from build123d import *

# Parameters (mm, degrees)
SKETCH1_R           = 8.743447226
SKETCH1_R_2         = 3
SKETCH1_R_3         = 10.172294787
SKETCH1_W           = 3
SKETCH1_H           = 12
BOSS_EXTRUDE1_DEPTH = 5
FILLET3_R           = 20
FILLET4_R           = 20
FILLET5_R           = 20


with BuildPart() as part:
    # Sketch1 → Boss-Extrude1 (new body)
    with BuildSketch(Plane(origin=(0, 0, 0), x_dir=(1, 0, 0), z_dir=(0, 1, 0))):
        Polygon((25, 35), (125, 35), (125, 111), (122, 111), (122, 123), (125, 123), (125, 175), (150, 175), (150, 200), (0, 200), (0, 175), (25, 175), (25, 123), (28, 123), (28, 111), (25, 111), align=None)
        with Locations(Location((75, 139.799864951, 0), (0, 0, 270))):
            Circle(SKETCH1_R, mode=Mode.SUBTRACT)
        with Locations(Location((93.745998674, 100, 0), (0, 0, 270))):
            Circle(SKETCH1_R_2, mode=Mode.SUBTRACT)
        with Locations(Location((93.745998674, 63.5, 0), (0, 0, 270))):
            Circle(SKETCH1_R_2, mode=Mode.SUBTRACT)
        with Locations(Location((75, 80.674864151, 0), (0, 0, 270))):
            Circle(SKETCH1_R_3, mode=Mode.SUBTRACT)
        with Locations(Location((57.245998674, 63.5, 0), (0, 0, 270))):
            Circle(SKETCH1_R_2, mode=Mode.SUBTRACT)
        with Locations(Location((57.245998674, 100, 0), (0, 0, 270))):
            Circle(SKETCH1_R_2, mode=Mode.SUBTRACT)
        with Locations((48, 117)):
            Rectangle(SKETCH1_W, SKETCH1_H, mode=Mode.SUBTRACT)
        with Locations(Location((45.771721368, 146.237160755, 0), (0, 0, 270))):
            Circle(SKETCH1_R_2, mode=Mode.SUBTRACT)
        with Locations(Location((45.771721368, 169.237160755, 0), (0, 0, 270))):
            Circle(SKETCH1_R_2, mode=Mode.SUBTRACT)
        with Locations((102, 117)):
            Rectangle(SKETCH1_W, SKETCH1_H, mode=Mode.SUBTRACT)
        with Locations(Location((103.771721368, 146.237160755, 0), (0, 0, 270))):
            Circle(SKETCH1_R_2, mode=Mode.SUBTRACT)
        with Locations(Location((103.771721368, 169.237160755, 0), (0, 0, 270))):
            Circle(SKETCH1_R_2, mode=Mode.SUBTRACT)
    extrude(amount=BOSS_EXTRUDE1_DEPTH)

    # Fillet3
    fillet3_edges = [part.edges().sort_by_distance(p)[0] for p in [
        (0, 2.5, -200),
    ]]
    fillet(fillet3_edges, radius=FILLET3_R)

    # Fillet4
    fillet4_edges = [part.edges().sort_by_distance(p)[0] for p in [
        (150, 2.5, -200),
    ]]
    fillet(fillet4_edges, radius=FILLET4_R)

    # Fillet5
    fillet5_edges = [part.edges().sort_by_distance(p)[0] for p in [
        (125, 2.5, -35),
        (25, 2.5, -35),
    ]]
    fillet(fillet5_edges, radius=FILLET5_R)


solid = part.part
Check sheet for the modelled part. Datum: model origin and axes. Units: mm. A direction names the side the tool comes from. Give positions to 0.01 mm unless a question says otherwise; leave off trailing zeros. Write each loop counter-clockwise with the first axis right and the second up, starting at its lowest first coordinate (ties: lowest second). Pieces come first, ordered by that corner, then holes. Notation, with made-up numbers: (24, 5.25) -> (80, 5.25) arc R18 ccw to (80, 14.25) -> close; hole circle Ø11 at (-9.75, -39.5). An arc over 180 degrees is marked (long way). Use one line per item in the form item = value. Start each with the question number.
1. Section check A-A (x = 75). Record the cut outline in (y, z).
2. Thickness scan on line 1 along X through (y, z) = (1.2, -100); line 2 along X through (y, z) = (2.25, -120); line 3 along Z through (x, y) = (69, 4.45). Record the ranges inside material, lowest first. Write a range as from..to.
3. Section check B-B (z = -100). Record the cut outline in (x, y), and give its area (3 significant figures).
4. Access from +Z, -Z, +X, -X, +Y, -Y to the whole of each face (thin tool, end or side, straight path). Record for faces 4 (the flat face through (28, 2, -117)), 5 (the flat face through (100.5, 2, -117)), 6 (the flat face through (125, 2, -83)), 7 (the flat face through (75, 2, -35)), 8 (the flat face through (76, 2, -200)).
5. Mould release check, pull along Z, two halves, no side actions. Record for faces 1 (the cylindrical face through (48.3, 2.46, -167.62)), 2 (the cylindrical face through (30.703, 2.535, -41.014)), 3 (the flat face through (74, 5, -119)): pulls with the +Z half, pulls with the -Z half, needs draft (parallel to the pull), parting line crosses it, or undercut.
6. Section check C-C (y = 1.95). Count the separate pieces of the cut face and the enclosed holes in it, and give its area (3 significant figures).
7. Go/stop test with flat-tipped pins: P1, Ø1.5, axis at y = 2, z = -128, coming from the +X side; P2, Ø1.5, axis at y = 3, z = -155, coming from the -X side; P3, Ø2.5, axis at x = 141.5, y = 3, coming from the +Z side. Record where each tip stops, or that it passes through.
Conclusion:
q1.outline = (0, -200) -> (5, -200) -> (5, -148.54) -> (0, -148.54) -> close; (0, -131.06) -> (5, -131.06) -> (5, -90.85) -> (0, -90.85) -> close; (0, -70.5) -> (5, -70.5) -> (5, -35) -> (0, -35) -> close
q2.line_1 = 25..54.25, 60.25..90.75, 96.75..125
q2.line_2 = 28..46.5, 49.5..100.5, 103.5..122
q2.line_3 = -200..-146.16, -133.44..-88.89, -72.46..-35
q3.outline = (25, 0) -> (54.25, 0) -> (54.25, 5) -> (25, 5) -> close; (60.25, 0) -> (90.75, 0) -> (90.75, 5) -> (60.25, 5) -> close; (96.75, 0) -> (125, 0) -> (125, 5) -> (96.75, 5) -> close
q3.area = 440 mm²
q4.face_4 = -X, +Y, -Y
q4.face_5 = +Y, -Y
q4.face_6 = +Z, +X, +Y, -Y
q4.face_7 = +Z, +X, -X, +Y, -Y
q4.face_8 = -Z, +X, -X, +Y, -Y
q5.face_1 = undercut
q5.face_2 = pulls with the +Z half
q5.face_3 = needs draft
q6.separate_pieces = 1
q6.enclosed_holes = 12
q6.area = 16,500 mm²
q7.P1 = 125
q7.P2 = 25
q7.P3 = -175
